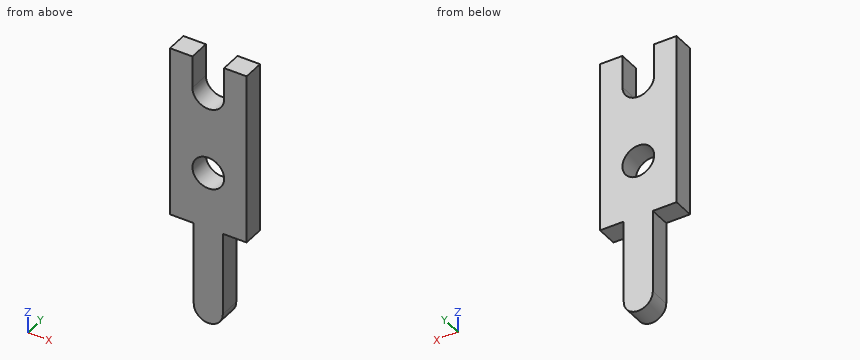
```python
from build123d import *

# Parameters (mm, degrees)
SKETCH_R  = 0.6
PAD_DEPTH = 0.4


with BuildPart() as part:
    # Sketch → Pad (new body, symmetric)
    with BuildSketch(Plane(origin=(0, 0, 0), x_dir=(-1, 0, 0), z_dir=(0, 1, 0))):
        with BuildLine():
            Line((-1.45, 6.5), (-1.45, 0))
            Line((-1.45, 0), (-0.55, 0))
            Line((-0.55, 0), (-0.55, -3.15))
            ThreePointArc((-0.55, -3.15), (0, -3.7), (0.55, -3.15))
            Line((0.55, 0), (0.55, -3.15))
            Line((0.55, 0), (1.45, 0))
            Line((1.45, 0), (1.45, 6.5))
            Line((1.45, 6.5), (0.6, 6.5))
            Line((0.6, 6.5), (0.6, 5.275))
            ThreePointArc((-0.6, 5.275), (0, 4.675), (0.6, 5.275))
            Line((-0.6, 5.275), (-0.6, 6.5))
            Line((-0.6, 6.5), (-1.45, 6.5))
        make_face()
        with Locations((0, 2.16645)):
            Circle(SKETCH_R, mode=Mode.SUBTRACT)
    extrude(amount=PAD_DEPTH, both=True)


solid = part.part
```
Part model, mm, in its own coordinate system. Give positions to 0.01 mm unless a question says otherwise; leave off trailing zeros. Write each loop counter-clockwise with the first axis right and the second up, starting at its lowest first coordinate (ties: lowest second). Pieces come first, ordered by that corner, then holes. Notation, with made-up numbers: M 81,-10.75 L 120,-10.75 A21 ccw 120,18.25 Z; hole C -21,43.5 d6. An arc over 180 degrees is marked long. Use CSV: the item, a comma, the result in double quotes.
Item 1: Slice it at A-A on x = 0. Write the cut outline in (y, z) (3 decimals).
Taken from the geometry:
outline,"M -0.4,-3.7 L 0.4,-3.7 L 0.4,1.566 L -0.4,1.566 Z; M -0.4,2.766 L 0.4,2.766 L 0.4,4.675 L -0.4,4.675 Z"
Item 2: Slice it at C-C on y = 0.05. Write the cut outline in (x, z) (3 decimals).
Taken from the geometry:
outline,"M -1.45,0 L -0.55,0 L -0.55,-3.15 A0.55 ccw 0.55,-3.15 L 0.55,0 L 1.45,0 L 1.45,6.5 L 0.6,6.5 L 0.6,5.275 A0.6 cw -0.6,5.275 L -0.6,6.5 L -1.45,6.5 Z; hole C 0,2.166 d1.2"
Item 3: Slice it at D-D on x = 0.8. Write the cut outline in (y, z), plus the area to 3 significant figures.
Taken from the geometry:
outline,"M -0.4,0 L 0.4,0 L 0.4,6.5 L -0.4,6.5 Z"
area,"5.20 mm²"
Item 4: Drill centre lines: probe 1 along Z at (x, y) = (0, -0.1) (3 decimals); probe 2 along X at (y, z) = (-0.3, 5.25); probe 3 along Z at (x, y) = (-0.75, -0.25). Where is each one in solid material? Low to high.
Taken from the geometry:
probe 1,"z = -3.7 to 1.566, 2.766 to 4.675"
probe 2,"x = -1.45 to -0.6, 0.6 to 1.45"
probe 3,"z = 0 to 6.5"
Item 5: Slice it at B-B on z = 5.75. Write the cut outline in (x, y), plus the area to 3 significant figures.
Taken from the geometry:
outline,"M -1.45,-0.4 L -0.6,-0.4 L -0.6,0.4 L -1.45,0.4 Z; M 0.6,-0.4 L 1.45,-0.4 L 1.45,0.4 L 0.6,0.4 Z"
area,"1.36 mm²"
Item 6: Pin check, flat tip, straight feed: P1, Ø0.7, axis at x = 0, z = 2.17, coming from the +Y side. Stop position of the tip, or through.
Taken from the geometry:
P1,"passes through"
